Autodesk Inventor part; units mm, degrees
ref_plane "YZ Plane" through (0, 0, 0) normal (1, 0, 0) x (0, 1, 0)
ref_plane "XZ Plane" through (0, 0, 0) normal (0, 1, 0) x (-1, 0, 0)
ref_plane "XY Plane" through (0, 0, 0) normal (0, 0, 1) x (1, 0, 0)
sketch "Sketch1" plane through (0, 0, 0) normal (0, 1, 0) x (-1, 0, 0)
  line L0 (-17.5, -17.5) -> (17.5, -17.5)
  line L1 (17.5, -17.5) -> (17.5, 17.5)
  line L2 (17.5, 17.5) -> (-17.5, 17.5)
  line L3 (-17.5, 17.5) -> (-17.5, -17.5)
  line L4 (-17.5, -17.5) -> (17.5, 17.5) construction
  line L5 (17.5, -17.5) -> (-17.5, 17.5) construction
  point P0 (0, 0)
  dimension "d0" = 35
  dimension "d1" = 35
extrude "Extrusion1" add sketch "Sketch1" along normal blind 15
sketch "Sketch2" plane through (0, 15, 0) normal (0, 1, 0) x (1, 0, 0)
  circle A0 centre (15, -15) radius 1
  circle A1 centre (-15, -15) radius 1
  circle A2 centre (15, 15) radius 1
  point P0 (0, 0)
  dimension "d10" = 2
  dimension "d11" = 15
  dimension "d12" = 15
  dimension "d13" = 2
  dimension "d14" = 15
  dimension "d15" = 15
  dimension "d16" = 2
  dimension "d17" = 15
  dimension "d18" = 15
extrude "Extrusion2" cut sketch "Sketch2" against normal blind 15
sketch "Sketch3" plane through (17.5, 0, -17.5) normal (0, 0, -1) x (-1, 0, 0)
  line L0 (0, 0) -> (0, 15)
  line L1 (35, 0) -> (35, 15)
  line L2 (0, 15) -> (35, 15)
  line L3 (35, 15) -> (35, 7.5)
  line L4 (35, 7.5) -> (0, 7.5)
  line L5 (0, 7.5) -> (0, 15)
  point P0 (17.5, 0)
extrude "Extrusion3" add sketch "Sketch3" along normal blind 9
sketch "Sketch4" plane through (-17.5, 0, 17.5) normal (0, 0, 1) x (1, 0, 0)
  line L0 (0, 15) -> (35, 15)
  line L1 (0, 7.5) -> (35, 7.5)
  line L2 (0, 15) -> (35, 15)
  line L3 (35, 15) -> (35, 7.5)
  line L4 (35, 7.5) -> (0, 7.5)
  line L5 (0, 7.5) -> (0, 15)
  point P0 (17.5, 0)
extrude "Extrusion4" add sketch "Sketch4" along normal blind 9
sketch "Sketch5" plane through (0, 15, 0) normal (0, 1, 0) x (1, 0, 0)
  circle A0 centre (4.5, -15.5) radius 1.25
  line L0 (-17.5, -26.5) -> (-17.5, 26.5)
  line L1 (-17.5, 0) -> (17.5, 0)
  line L2 (17.5, 26.5) -> (17.5, -26.5)
  line L3 (0, -26.5) -> (0, 26.5)
  line L4 (-26.5, 0) -> (8.5, 0)
  circle A1 centre (-4.5, -15.5) radius 1.25
  line L5 (-17.5, 31) -> (17.5, 31)
  circle A2 centre (4.5, 15.5) radius 1.25
  line L6 (-26.5, 31) -> (8.5, 31)
  circle A3 centre (-4.5, 15.5) radius 1.25
  point P0 (0, 0)
  dimension "d25" = 15.5
  dimension "d26" = 4.5
  dimension "d27" = 2.5
  dimension "d30" = 9
  dimension "d33" = 31
extrude "Extrusion5" cut sketch "Sketch5" against normal blind 2
properties part number "actuator"
Part model, mm, in its own coordinate system. A direction names the side the tool comes from. Round coordinates to 2 decimals unless told otherwise and drop trailing zeros. Write each loop counter-clockwise with the first axis right and the second up, starting at its lowest first coordinate (ties: lowest second). Pieces come first, ordered by that corner, then holes. Notation, with made-up numbers: (52.5, 80.25) - (64.5, 80.25) arc R16 ccw to (64.5, 86.25) - close; hole circle Ø8 at (-21, -30.5). An arc over 180 degrees is marked (long way). Use CSV: the item, a comma, the result in double quotes.
Item 1: Tool access for faces 1 (the flat face through (0, 7.5, -22)), 2 (the flat face through (0, 4, 17.5)), 3 (the flat face through (0, 15, 0)), 4 (the cylindrical face through (15, 8, -14)), 5 (the flat face through (-5, 13, -16)): list every direction of +Z, -Z, +X, -X, +Y, -Y with a clear straight run to the whole face (end or side of a thin tool).
Results list:
face 1,"-Z, +X, -X, -Y"
face 2,"+Z, +X, -X, -Y"
face 3,"+Z, -Z, +X, -X, +Y"
face 4,"+Y, -Y"
face 5,"+Y"
Item 2: Slice it at D-D, the plane x = 4.5. Write the cut outline in (y, z).
Results list:
outline,"(0, -17.5) - (7.5, -17.5) - (7.5, -26.5) - (15, -26.5) - (15, -16.75) - (13, -16.75) - (13, -14.25) - (15, -14.25) - (15, 14.25) - (13, 14.25) - (13, 16.75) - (15, 16.75) - (15, 26.5) - (7.5, 26.5) - (7.5, 17.5) - (0, 17.5) - close"
Item 3: Slice it at C-C, the plane x = -15. Write the cut outline in (y, z), then the cut area to 3 significant figures.
Results list:
outline,"(0, -17.5) - (7.5, -17.5) - (7.5, -26.5) - (15, -26.5) - (15, 14) - (0, 14) - close; (0, 16) - (15, 16) - (15, 26.5) - (7.5, 26.5) - (7.5, 17.5) - (0, 17.5) - close"
area,"630 mm²"
Item 4: Pull direction X, two halves, no side cores. Call faces 6 (the flat face through (17.5, 8, 0)), 7 (the flat face through (-17.5, 7, 0)), 8 (the flat face through (0, 11, -26.5)), 9 (the cylindrical face through (-3.828, 14.014, -16.554)): pulls with the +X half, pulls with the -X half, needs draft (parallel to the pull), parting line crosses it, or undercut.
Results list:
face 6,"pulls with the +X half"
face 7,"pulls with the -X half"
face 8,"needs draft"
face 9,"undercut"
Item 5: Slice it at A-A, the plane x = 15. Write the cut outline in (y, z), then the cut area to 3 significant figures.
Results list:
outline,"(0, -17.5) - (7.5, -17.5) - (7.5, -26.5) - (15, -26.5) - (15, -16) - (0, -16) - close; (0, -14) - (15, -14) - (15, 14) - (0, 14) - close; (0, 16) - (15, 16) - (15, 26.5) - (7.5, 26.5) - (7.5, 17.5) - (0, 17.5) - close"
area,"600 mm²"
Item 6: Wall check: L1, parallel to X at y = 9.5, z = 15; L2, parallel to Z at x = -4.5, y = 13.8; L3, parallel to Z at x = -15, y = 4. Give the ranges that are in metal, low to high.
Results list:
L1,"x = -17.5 to -16, -14 to 14, 16 to 17.5"
L2,"z = -26.5 to -16.75, -14.25 to 14.25, 16.75 to 26.5"
L3,"z = -17.5 to 14, 16 to 17.5"
Item 7: Flat gauge pins, fed straight in: P1, Ø2, axis at x = 4.5, z = 15.5, coming from the +Y side; P2, Ø4, axis at x = 1.5, y = 4, coming from the +Z side; P3, Ø2, axis at x = -5, y = 4.5, coming from the -Z side. Where does each tip first touch, or does it go through?
Results list:
P1,"stops at y = 13"
P2,"stops at z = 17.5"
P3,"stops at z = -17.5"
Item 8: Slice it at B-B, the plane y = 6. Write the cut outline in (x, z).
Results list:
outline,"(-17.5, -17.5) - (17.5, -17.5) - (17.5, 17.5) - (-17.5, 17.5) - close; hole circle Ø2 at (-15, 15); hole circle Ø2 at (15, -15); hole circle Ø2 at (15, 15)"
